from build123d import *
from build123d.topology import SkipClean

# Parameters (mm, degrees)
SKETCH_1_R          = 17.5
EXTRUDE_1_DEPTH     = 3
EXTRUDE_START       = -20
EXTRUDE_2_DEPTH     = 20
SKETCH_3_W          = 42.038336367
SKETCH_3_H          = 17.5
CUT_EXTRUDE_2_DEPTH = 17
FILLET_1_R          = 0.8
SKETCH_4_R          = 5.5
CUT_EXTRUDE_3_DEPTH = 32.547583109
SKETCH_5_R          = 5.5
EXTRUDE_3_DEPTH     = 3.5
CUT_EXTRUDE_START   = -3.5
CUT_EXTRUDE_5_DEPTH = 3.5
CUT_EXTRUDE_6_DEPTH = 6.5


with BuildPart() as part:
    # 草图1 → 凸台-拉伸1 (new body)
    with BuildSketch(Plane.XY):
        Circle(SKETCH_1_R)
        with BuildLine():
            Line((1.6, 14.5), (1.6, 10.5))
            ThreePointArc((1.6, 10.5), (0, 8.9), (-1.6, 10.5))
            Line((-1.6, 10.5), (-1.6, 14.5))
            ThreePointArc((-1.6, 14.5), (0, 16.1), (1.6, 14.5))
        make_face(mode=Mode.SUBTRACT)
        with BuildLine():
            Line((1.6, -14.5), (1.6, -10.5))
            ThreePointArc((1.6, -10.5), (0, -8.9), (-1.6, -10.5))
            Line((-1.6, -10.5), (-1.6, -14.5))
            ThreePointArc((-1.6, -14.5), (0, -16.1), (1.6, -14.5))
        make_face(mode=Mode.SUBTRACT)
        with BuildLine():
            Line((-12, 1.6), (-8, 1.6))
            ThreePointArc((-8, 1.6), (-6.4, 0), (-8, -1.6))
            Line((-8, -1.6), (-12, -1.6))
            ThreePointArc((-12, -1.6), (-13.6, 0), (-12, 1.6))
        make_face(mode=Mode.SUBTRACT)
        with BuildLine():
            Line((12, 1.6), (8, 1.6))
            ThreePointArc((8, 1.6), (6.4, 0), (8, -1.6))
            Line((8, -1.6), (12, -1.6))
            ThreePointArc((12, -1.6), (13.6, 0), (12, 1.6))
        make_face(mode=Mode.SUBTRACT)
    extrude(amount=EXTRUDE_1_DEPTH)

    # 草图2 → 凸台-拉伸2 (add)
    with BuildSketch(Plane.XY.offset(3).offset(EXTRUDE_START)):
        with BuildLine():
            Line((-17.5, -20), (17.5, -20))
            Line((17.5, -20), (17.5, 0))
            ThreePointArc((17.5, 0), (0, -17.5), (-17.5, 0))
            Line((-17.5, 0), (-17.5, -20))
        make_face()
    extrude(amount=EXTRUDE_2_DEPTH)

    # 草图3 → 切除-拉伸2 (cut)
    with BuildSketch(Plane(origin=(0, 0, -17), x_dir=(-1, 0, 0), z_dir=(0, 0, -1))):
        with Locations((-0.801424091, -8.75)):
            Rectangle(SKETCH_3_W, SKETCH_3_H)
    extrude(amount=-CUT_EXTRUDE_2_DEPTH, mode=Mode.SUBTRACT)

    # 圆角1
    fillet_1_edges = [part.edges().sort_by_distance(p)[0] for p in [
        (17.5, -18.75, -17),
        (0, -20, -17),
        (-17.5, -18.75, -17),
        (0, -17.5, 0),
    ]]
    fillet(fillet_1_edges, radius=FILLET_1_R)

    # 草图4 → 切除-拉伸3 (cut, through all)
    with BuildSketch(Plane(origin=(0, 0, 0), x_dir=(-1, 0, 0), z_dir=(0, 0, -1))):
        Circle(SKETCH_4_R)
    extrude(amount=-CUT_EXTRUDE_3_DEPTH, mode=Mode.SUBTRACT)

    # 草图5 → 凸台-拉伸3 (add)
    with SkipClean():  # the faces are left unmerged after this step: merging them gives an invalid solid
        with BuildSketch(Plane.XY.offset(3)):
            with BuildLine():
                Line((-17.5, 0), (-17.5, -20))
                Line((-17.5, -20), (17.5, -20))
                Line((17.5, -20), (17.5, 0))
                ThreePointArc((17.5, 0), (0, 17.5), (-17.5, 0))
            make_face()
            with Locations(Location((0, 0, 0), (0, 0, 180))):
                Circle(SKETCH_5_R, mode=Mode.SUBTRACT)
            with BuildLine():
                Line((1.6, -14.5), (1.6, -10.5))
                ThreePointArc((1.6, -10.5), (0, -8.9), (-1.6, -10.5))
                Line((-1.6, -10.5), (-1.6, -14.5))
                ThreePointArc((-1.6, -14.5), (0, -16.1), (1.6, -14.5))
            make_face(mode=Mode.SUBTRACT)
            with BuildLine():
                Line((-8, 1.6), (-12, 1.6))
                ThreePointArc((-12, 1.6), (-13.6, 0), (-12, -1.6))
                Line((-12, -1.6), (-8, -1.6))
                ThreePointArc((-8, -1.6), (-6.4, 0), (-8, 1.6))
            make_face(mode=Mode.SUBTRACT)
            with BuildLine():
                Line((8, -1.6), (12, -1.6))
                ThreePointArc((12, -1.6), (13.6, 0), (12, 1.6))
                Line((12, 1.6), (8, 1.6))
                ThreePointArc((8, 1.6), (6.4, 0), (8, -1.6))
            make_face(mode=Mode.SUBTRACT)
            with BuildLine():
                Line((1.6, 10.5), (1.6, 14.5))
                ThreePointArc((1.6, 14.5), (0, 16.1), (-1.6, 14.5))
                Line((-1.6, 14.5), (-1.6, 10.5))
                ThreePointArc((-1.6, 10.5), (0, 8.9), (1.6, 10.5))
            make_face(mode=Mode.SUBTRACT)
        extrude(amount=EXTRUDE_3_DEPTH)
    add(part.part.scale(1), mode=Mode.REPLACE)  # the faces are merged on a copy

    # 草图7 → 切除-拉伸5 (cut)
    # profile 1 of 4: a face of its own
    with BuildSketch(Plane.XY.offset(6.5).offset(CUT_EXTRUDE_START)):
        with BuildLine():
            Line((2.8, -14.5), (2.8, -10.5))
            ThreePointArc((2.8, -10.5), (0, -7.7), (-2.8, -10.5))
            Line((-2.8, -10.5), (-2.8, -14.5))
            ThreePointArc((-2.8, -14.5), (0, -17.3), (2.8, -14.5))
        make_face()
        with BuildLine():
            Line((1.6, -14.5), (1.6, -10.5))
            ThreePointArc((1.6, -10.5), (0, -8.9), (-1.6, -10.5))
            Line((-1.6, -10.5), (-1.6, -14.5))
            ThreePointArc((-1.6, -14.5), (0, -16.1), (1.6, -14.5))
        make_face(mode=Mode.SUBTRACT)
    # profile 2 of 4: a face of its own
    with BuildSketch(Plane.XY.offset(6.5).offset(CUT_EXTRUDE_START)):
        with BuildLine():
            Line((8, -2.8), (12, -2.8))
            ThreePointArc((12, -2.8), (14.8, 0), (12, 2.8))
            Line((12, 2.8), (8, 2.8))
            ThreePointArc((8, 2.8), (5.2, 0), (8, -2.8))
        make_face()
        with BuildLine():
            Line((8, -1.6), (12, -1.6))
            ThreePointArc((12, -1.6), (13.6, 0), (12, 1.6))
            Line((12, 1.6), (8, 1.6))
            ThreePointArc((8, 1.6), (6.4, 0), (8, -1.6))
        make_face(mode=Mode.SUBTRACT)
    # profile 3 of 4: a face of its own
    with BuildSketch(Plane.XY.offset(6.5).offset(CUT_EXTRUDE_START)):
        with BuildLine():
            Line((-12, -2.8), (-8, -2.8))
            ThreePointArc((-8, -2.8), (-5.2, 0), (-8, 2.8))
            Line((-8, 2.8), (-12, 2.8))
            ThreePointArc((-12, 2.8), (-14.8, 0), (-12, -2.8))
        make_face()
        with BuildLine():
            Line((-12, -1.6), (-8, -1.6))
            ThreePointArc((-8, -1.6), (-6.4, 0), (-8, 1.6))
            Line((-8, 1.6), (-12, 1.6))
            ThreePointArc((-12, 1.6), (-13.6, 0), (-12, -1.6))
        make_face(mode=Mode.SUBTRACT)
    # profile 4 of 4: a face of its own
    with BuildSketch(Plane.XY.offset(6.5).offset(CUT_EXTRUDE_START)):
        with BuildLine():
            Line((2.8, 10.5), (2.8, 14.5))
            ThreePointArc((2.8, 14.5), (0, 17.3), (-2.8, 14.5))
            Line((-2.8, 14.5), (-2.8, 10.5))
            ThreePointArc((-2.8, 10.5), (0, 7.7), (2.8, 10.5))
        make_face()
        with BuildLine():
            Line((1.6, 10.5), (1.6, 14.5))
            ThreePointArc((1.6, 14.5), (0, 16.1), (-1.6, 14.5))
            Line((-1.6, 14.5), (-1.6, 10.5))
            ThreePointArc((-1.6, 10.5), (0, 8.9), (1.6, 10.5))
        make_face(mode=Mode.SUBTRACT)
    extrude(amount=CUT_EXTRUDE_5_DEPTH, mode=Mode.SUBTRACT)

    # 草图8 → 切除-拉伸6 (cut)
    with BuildSketch(Plane.XY.offset(6.5)):
        with BuildLine():
            Line((11.561195872, 9.298454173), (8.379215357, 6.116473657))
            ThreePointArc((8.379215357, 6.116473657), (6.116473657, 6.116473657), (6.116473657, 8.379215357))
            Line((6.116473657, 8.379215357), (9.298454173, 11.561195872))
            ThreePointArc((9.298454173, 11.561195872), (11.561195872, 11.561195872), (11.561195872, 9.298454173))
        make_face()
        with BuildLine():
            Line((-8.379215357, 6.116473657), (-11.561195872, 9.298454173))
            ThreePointArc((-11.561195872, 9.298454173), (-11.561195872, 11.561195872), (-9.298454173, 11.561195872))
            Line((-9.298454173, 11.561195872), (-6.116473657, 8.379215357))
            ThreePointArc((-6.116473657, 8.379215357), (-6.116473657, 6.116473657), (-8.379215357, 6.116473657))
        make_face()
        with BuildLine():
            Line((6.116473657, -8.379215357), (9.298454173, -11.561195872))
            ThreePointArc((9.298454173, -11.561195872), (11.561195872, -11.561195872), (11.561195872, -9.298454173))
            Line((11.561195872, -9.298454173), (8.379215357, -6.116473657))
            ThreePointArc((8.379215357, -6.116473657), (6.116473657, -6.116473657), (6.116473657, -8.379215357))
        make_face()
        with BuildLine():
            Line((-9.298454173, -11.561195872), (-6.116473657, -8.379215357))
            ThreePointArc((-6.116473657, -8.379215357), (-6.116473657, -6.116473657), (-8.379215357, -6.116473657))
            Line((-8.379215357, -6.116473657), (-11.561195872, -9.298454173))
            ThreePointArc((-11.561195872, -9.298454173), (-11.561195872, -11.561195872), (-9.298454173, -11.561195872))
        make_face()
    extrude(amount=-CUT_EXTRUDE_6_DEPTH, mode=Mode.SUBTRACT)


solid = part.part
Input: part model. Units: mm. Frame: model coordinates. A direction names the side the tool comes from. Give positions to 0.01 mm unless a question says otherwise; leave off trailing zeros. Loops run counter-clockwise (first coordinate to the right, second up) from the corner with the lowest first, then second, coordinate; pieces in that order, holes last. Notation, with made-up numbers: M -1.75,49 L 3.25,49 A17 cw 3.25,61 Z; hole C 15.5,-38 d6. An arc over 180 degrees is marked long. Use one line per item in the form item = value.
1. Reachability of faces 3 (the face through (0, 16.1, 1.5)), 4 (the face through (10, -2.8, 5)) from +Z, -Z, +X, -X, +Y, -Y: full face, straight path, thin tool, end or side. Return the list, or none.
Numbers:
face_3 = +Z, -Z
face_4 = +Z
2. Section query D-D, the plane z = -14.5. Return the cut outline in (x, y), and give its area (3 significant figures).
Numbers:
outline = M -17.5,-20 L 17.5,-20 L 17.5,-17.5 L -17.5,-17.5 Z
area = 87.5 mm²
3. Section query B-B, the plane y = 15.5. Return the cut outline in (x, z), and give its area (3 significant figures).
Numbers:
outline = M -8.12,0 L -1.25,0 L -1.25,3 L -2.62,3 L -2.62,6.5 L -8.12,6.5 Z; M 1.25,0 L 8.12,0 L 8.12,6.5 L 2.62,6.5 L 2.62,3 L 1.25,3 Z
area = 79.8 mm²
4. Section query C-C, the plane z = 2.5. Count the separate pieces of the cut face and the enclosed holes in it, and give its area (3 significant figures).
Numbers:
separate_pieces = 1
enclosed_holes = 9
area = 913 mm²
5. Pull-direction query (Y, two-part tool) for faces 1 (the face through (-4, -5, 6.5)), 2 (the face through (-6.4, 2.3, 4.7)); classes: released by +Y, released by -Y, zero draft, split by the parting line, or undercut.
Numbers:
face_1 = zero draft
face_2 = undercut
6. Section query A-A, the plane x = 0. Return the cut outline in (y, z), and give its area (3 significant figures).
Numbers:
outline = M -20,-16.2 A0.8 ccw -19.2,-17 L -17.5,-17 L -17.5,-0.8 A0.8 cw -16.7,0 L -16.1,0 L -16.1,3 L -17.3,3 L -17.3,6.5 L -20,6.5 Z; M -8.9,0 L -5.5,0 L -5.5,6.5 L -7.7,6.5 L -7.7,3 L -8.9,3 Z; M 5.5,0 L 8.9,0 L 8.9,3 L 7.7,3 L 7.7,6.5 L 5.5,6.5 Z; M 16.1,0 L 17.5,0 L 17.5,6.5 L 17.3,6.5 L 17.3,3 L 16.1,3 Z
area = 104 mm²
7. First-contact query: pin 1 (2.5 mm diameter, centred on y = 12.5, z = 2, fed in from -X); pin 2 (3.5 mm diameter, centred on x = -10.5, z = 1.5, fed in from +Y); pin 3 (17.5 mm diameter, centred on x = 0, y = 0, fed in from -Z); pin 4 (5 mm diameter, centred on x = 12, y = -15.5, fed in from -Z). Flat tips, straight axial feed; report the tip coordinate or a pass-through.
Numbers:
pin_1 = -13.4
pin_2 = 15.16
pin_3 = 0
pin_4 = -17
8. Line query: L1, parallel to Y at x = 0, z = 2.5; L2, parallel to Y at x = 0, z = 4; L3, parallel to X at y = -12.5, z = 5.25. Output: solid intervals per line, ascending.
Numbers:
L1 = -20 to -16.1, -8.9 to -5.5, 5.5 to 8.9, 16.1 to 17.5
L2 = -20 to -17.3, -7.7 to -5.5, 5.5 to 7.7, 17.3 to 17.5
L3 = -17.5 to -2.8, 2.8 to 17.5
